Can you work these out from the model? Positions are in its coordinate system, mm. Face numbers are marked on the shaded views. A direction names the side the tool comes from. Give positions to 0.01 mm unless a question says otherwise; leave off trailing zeros. Order: outer loops, then holes, each group sorted by start corner. A loop starts at its lowest first (then second) coordinate and runs counter-clockwise, first axis right, second up.
Item 1: If we mould it in two halves opening along X, with no side actions, what happens to the marked faces 1, 2, 3 and 4? For each: +X half, -X half, draft (parallel to the pull), parting line (faces both ways), or undercut.
Item 2: Which directions (+Z, -Z, +X, -X, +Y, -Y) give clear straight access to the entire face, cutting with the end or side of a thin tool? Please do the marked faces 5 and 6.
Item 3: I want a section at C-C, the plane y = -5. Write out the boundary of the cut face in (x, z), then the cut area to 3 significant figures.
Item 4: I want a section at A-A, the plane y = 0. Write out the boundary of the cut face in (x, z).
Item 5: If I drill on line 1 along Y through (x, z) = (0, 4.5); line 2 along Y through (x, z) = (2, -5.75); line 3 along Z through (x, y) = (-6, -11), over which ranges is the centre line in solid material (lowest first)?
Item 6: I want a section at D-D, the plane z = 5.5. Write out the boundary of the cut face in (x, y), then the cut area to 3 significant figures.
Item 7: I want a section at B-B, the plane x = 0. Write out the boundary of the cut face in (y, z), then the cut area to 3 significant figures.
Item 8: I'm going to push flat-ended pins straight in: pin 1 Ø5 at (x, z) = (-4.5, 5.5) entering from -Y; pin 2 Ø6 at (x, z) = (-5, 1) entering from +Y; pin 3 Ø3.5 at (y, z) = (-17.5, -3.5) entering from -X. Where does each tip first touch, or does it pass through?
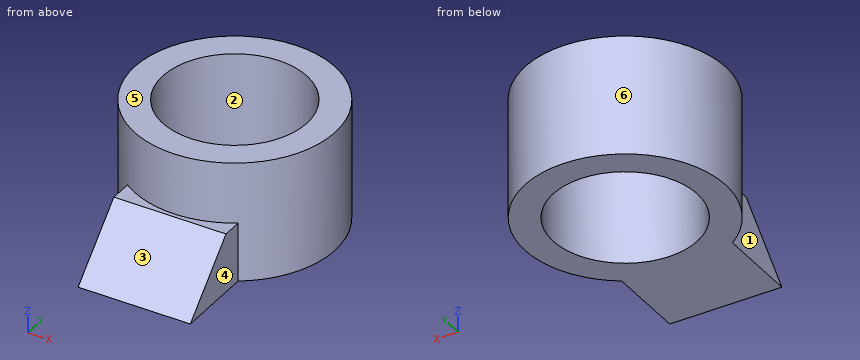
```python
from build123d import *

# Parameters (mm, degrees)
F0_R        = 12.5
F1_DEPTH    = 7.5
F2_R        = 9
F3_DEPTH    = 25
F4_W        = 14
F4_H        = 7.3697703017
F5_DEPTH    = 23
F6_R        = 9
F7_DEPTH    = 25
F8_T1_DEPTH = 65.4336597593


# Not quite as in the source:
# - a fillet or chamfer that OpenCascade refuses, or shapes differently, is made with other operations: its cross-section is extruded or revolved along the edge and cut away or added


with BuildPart() as f1:
    # F0 (on Top) → F1 (new body, symmetric)
    with BuildSketch(Plane.XY):
        Circle(F0_R)
    extrude(amount=F1_DEPTH, both=True)

    # F2 (on face) → F3 (cut)
    with BuildSketch(Plane.XY.offset(7.5)):
        Circle(F2_R)
    extrude(amount=-F3_DEPTH, mode=Mode.SUBTRACT)

    # F4 (on Front) → F5 (join)
    with BuildSketch(Plane.XZ):
        with Locations((-0.2285402901, -3.8151148492)):
            Rectangle(F4_W, F4_H)
    extrude(amount=F5_DEPTH)

    # F6 (on face) → F7 (cut)
    with BuildSketch(Plane(origin=(0, 0, -7.5), x_dir=(1, 0, 0), z_dir=(0, 0, -1))):
        Circle(F6_R)
    extrude(amount=-F7_DEPTH, mode=Mode.SUBTRACT)

    # F8: chamfer of 10 on 1 edges, made by hand

    # F8_s2 → F8_t1 (cut)
    with BuildSketch(Plane.YZ.offset(-32.9453701698)):
        Polygon((-23, -10.1302296983), (-13, -0.1302296983), (-23, -0.1302296983), align=None)
    extrude(amount=F8_T1_DEPTH, mode=Mode.SUBTRACT)


solid = f1.part
```
Results list:
1. face 1: -X half
1. face 2: undercut
1. face 3: draft
1. face 4: +X half
2. face 5: +Z, +X, -X, +Y, -Y
2. face 6: +Z
3. outline: (-11.46, -7.5) - (-7.48, -7.5) - (-7.48, 7.5) - (-11.46, 7.5) - close; (7.48, -7.5) - (11.46, -7.5) - (11.46, 7.5) - (7.48, 7.5) - close
3. area: 119 mm2
4. outline: (-12.5, -7.5) - (-9, -7.5) - (-9, 7.5) - (-12.5, 7.5) - close; (9, -7.5) - (12.5, -7.5) - (12.5, 7.5) - (9, 7.5) - close
5. line 1: y = -12.5 to -9, 9 to 12.5
5. line 2: y = -18.62 to -8.77, 8.77 to 12.34
5. line 3: z = -7.5 to -0.13
6. outline: circle Ø25 at (0, 0); hole circle Ø18 at (0, 0)
6. area: 236 mm2
7. outline: (-20.37, -7.5) - (-9, -7.5) - (-9, 7.5) - (-12.5, 7.5) - (-12.5, -0.13) - (-13, -0.13) - close; (9, -7.5) - (12.5, -7.5) - (12.5, 7.5) - (9, 7.5) - close
7. area: 136 mm2
8. pin 1: stops at y = -12.34
8. pin 2: stops at y = 12.34
8. pin 3: stops at x = -7.23
